Autodesk Fusion 360 part; units mm, degrees
sketch "Skizze1" plane through (0, 0, 0) normal (0, 0, 1) x (1, 0, 0)
  line L0 (-19, 19) -> (19, 19)
  line L1 (19, 19) -> (19, -19)
  line L2 (19, -19) -> (-19, -19)
  line L3 (-19, -19) -> (-19, 19)
  circle A0 centre (-14, 14) radius 1.175
  line L4 (0, 19) -> (0, -19) construction
  line L5 (-19, 0) -> (19, 0) construction
  circle A1 centre (14, 14) radius 1.175
  circle A2 centre (-14, -14) radius 1.175
  circle A3 centre (14, -14) radius 1.175
  circle A4 centre (-17, 17) radius 1
  circle A5 centre (17, 17) radius 1
  circle A6 centre (-17, -17) radius 1
  circle A7 centre (17, -17) radius 1
  circle A8 centre (-10, 0) radius 1
  circle A9 centre (10, 0) radius 1
  line L6 (-17, 16.5) -> (-6.5, 16.5) construction
  line L7 (-4.5, 16.5) -> (4.5, 16.5) construction
  line L8 (-4.5, 16) -> (4.5, 16)
  arc A10 (4.5, 16) -> (4.5, 17) centre (4.5, 16.5) ccw
  line L9 (4.5, 17) -> (-4.5, 17)
  arc A11 (-4.5, 17) -> (-4.5, 16) centre (-4.5, 16.5) ccw
  line L10 (-4.5, 16.5) -> (4.5, 16.5) construction
  line L11 (-6.5, 17) -> (-17, 17)
  arc A12 (-17, 17) -> (-17, 16) centre (-17, 16.5) ccw
  line L12 (-17, 16) -> (-6.5, 16)
  arc A13 (-6.5, 16) -> (-6.5, 17) centre (-6.5, 16.5) ccw
  line L13 (-6.5, 16.5) -> (-17, 16.5) construction
  line L14 (-19, 19) -> (19, -19) construction
  line L15 (6.5, 17) -> (17, 17)
  arc A14 (17, 16) -> (17, 17) centre (17, 16.5) ccw
  arc A15 (6.5, 17) -> (6.5, 16) centre (6.5, 16.5) ccw
  line L16 (17, 16) -> (6.5, 16)
  line L17 (-6.5, -17) -> (-17, -17)
  arc A16 (-17, -16) -> (-17, -17) centre (-17, -16.5) ccw
  arc A17 (-6.5, -17) -> (-6.5, -16) centre (-6.5, -16.5) ccw
  line L18 (4.5, -17) -> (-4.5, -17)
  arc A18 (-4.5, -16) -> (-4.5, -17) centre (-4.5, -16.5) ccw
  arc A19 (4.5, -17) -> (4.5, -16) centre (4.5, -16.5) ccw
  arc A20 (6.5, -16) -> (6.5, -17) centre (6.5, -16.5) ccw
  line L19 (6.5, -17) -> (17, -17)
  arc A21 (17, -17) -> (17, -16) centre (17, -16.5) ccw
  line L20 (17, -16) -> (6.5, -16)
  line L21 (-4.5, -16) -> (4.5, -16)
  line L22 (-17, -16) -> (-6.5, -16)
  line L23 (-17, -4.5) -> (-17, 4.5)
  arc A22 (-16, 4.5) -> (-17, 4.5) centre (-16.5, 4.5) ccw
  arc A23 (-17, -4.5) -> (-16, -4.5) centre (-16.5, -4.5) ccw
  line L24 (-16, 4.5) -> (-16, -4.5)
  arc A24 (17, 4.5) -> (16, 4.5) centre (16.5, 4.5) ccw
  line L25 (16, 4.5) -> (16, -4.5)
  arc A25 (16, -4.5) -> (17, -4.5) centre (16.5, -4.5) ccw
  line L26 (17, -4.5) -> (17, 4.5)
  line L27 (-17, 6.5) -> (-17, 17)
  arc A26 (-16, 17) -> (-17, 17) centre (-16.5, 17) ccw
  arc A27 (-17, 6.5) -> (-16, 6.5) centre (-16.5, 6.5) ccw
  line L28 (-16, 17) -> (-16, 6.5)
  arc A28 (-16, -6.5) -> (-17, -6.5) centre (-16.5, -6.5) ccw
  line L29 (-17, -6.5) -> (-17, -17)
  arc A29 (-17, -17) -> (-16, -17) centre (-16.5, -17) ccw
  line L30 (-16, -17) -> (-16, -6.5)
  arc A30 (17, 17) -> (16, 17) centre (16.5, 17) ccw
  line L31 (16, 17) -> (16, 6.5)
  arc A31 (16, 6.5) -> (17, 6.5) centre (16.5, 6.5) ccw
  line L32 (17, 6.5) -> (17, 17)
  line L33 (16, -17) -> (16, -6.5)
  arc A32 (17, -6.5) -> (16, -6.5) centre (16.5, -6.5) ccw
  arc A33 (16, -17) -> (17, -17) centre (16.5, -17) ccw
  line L34 (17, -6.5) -> (17, -17)
  dimension "d1" = 38
  dimension "d2" = 38
  dimension "d3" = 2.35
  dimension "d6" = 28
  dimension "d7" = 28
  dimension "d8" = 2
  dimension "d9" = 34
  dimension "d10" = 34
  dimension "d17" = 2
  dimension "d18" = 20
  dimension "d20" = 9
  dimension "d21" = 1
  dimension "d22" = 2
  dimension "d23" = 2.5
  dimension "d24" = 1
  dimension "d25" = 2
extrude "Extrusion1" add sketch "Skizze1" along normal blind 1.5
fillet "Abrundung1" radius 1 4 edges at (-16, -16, 0.75) (16, -16, 0.75) (16, 16, 0.75) (-16, 16, 0.75)
sketch "Skizze2" plane through (0, 0, 1.5) normal (0, 0, 1) x (-1, 0, 0)
  circle A0 centre (14, -14) radius 1.175
  circle A1 centre (-14, 14) radius 1.175
  circle A2 centre (14, 14) radius 1.175
  circle A3 centre (-14, -14) radius 1.175
  line L0 (19, 19) -> (-19, 19)
  line L1 (-19, 19) -> (-19, -19)
  line L2 (-19, -19) -> (19, -19)
  line L3 (19, -19) -> (19, 19)
  line L4 (8, -8) -> (-8, -8)
  line L5 (-8, -8) -> (-8, 8)
  line L6 (-8, 8) -> (8, 8)
  line L7 (8, 8) -> (8, -8)
  line L8 (0, -19) -> (0, 19) construction
  line L9 (19, 0) -> (-19, 0) construction
  circle A4 centre (10, 0) radius 1
  circle A5 centre (-10, 0) radius 1
  line L10 (-17, -4.5) -> (-17, 4.5)
  arc A6 (-16, 4.5) -> (-17, 4.5) centre (-16.5, 4.5) ccw
  line L11 (-16, 4.5) -> (-16, -4.5)
  arc A7 (-17, -4.5) -> (-16, -4.5) centre (-16.5, -4.5) ccw
  line L12 (-6.5, 16) -> (-15, 16)
  line L13 (-16, 15) -> (-16, 6.5)
  arc A8 (-17, 6.5) -> (-16, 6.5) centre (-16.5, 6.5) ccw
  line L14 (-17, 6.5) -> (-17, 16)
  arc A9 (-16, 17) -> (-17, 16) centre (-17, 17) ccw
  line L15 (-16, 17) -> (-6.5, 17)
  arc A10 (-6.5, 16) -> (-6.5, 17) centre (-6.5, 16.5) ccw
  arc A11 (-4.5, 17) -> (-4.5, 16) centre (-4.5, 16.5) ccw
  line L16 (-4.5, 17) -> (4.5, 17)
  arc A12 (4.5, 16) -> (4.5, 17) centre (4.5, 16.5) ccw
  line L17 (4.5, 16) -> (-4.5, 16)
  line L18 (-16, -6.5) -> (-16, -15)
  line L19 (-15, -16) -> (-6.5, -16)
  arc A13 (-6.5, -17) -> (-6.5, -16) centre (-6.5, -16.5) ccw
  line L20 (-6.5, -17) -> (-16, -17)
  arc A14 (-17, -16) -> (-16, -17) centre (-17, -17) ccw
  line L21 (-17, -16) -> (-17, -6.5)
  arc A15 (-16, -6.5) -> (-17, -6.5) centre (-16.5, -6.5) ccw
  line L22 (16, 6.5) -> (16, 15)
  line L23 (15, 16) -> (6.5, 16)
  arc A16 (6.5, 17) -> (6.5, 16) centre (6.5, 16.5) ccw
  line L24 (6.5, 17) -> (16, 17)
  arc A17 (17, 16) -> (16, 17) centre (17, 17) ccw
  line L25 (17, 16) -> (17, 6.5)
  arc A18 (16, 6.5) -> (17, 6.5) centre (16.5, 6.5) ccw
  arc A19 (17, 4.5) -> (16, 4.5) centre (16.5, 4.5) ccw
  line L26 (17, 4.5) -> (17, -4.5)
  arc A20 (16, -4.5) -> (17, -4.5) centre (16.5, -4.5) ccw
  line L27 (16, -4.5) -> (16, 4.5)
  arc A21 (4.5, -17) -> (4.5, -16) centre (4.5, -16.5) ccw
  line L28 (4.5, -17) -> (-4.5, -17)
  arc A22 (-4.5, -16) -> (-4.5, -17) centre (-4.5, -16.5) ccw
  line L29 (-4.5, -16) -> (4.5, -16)
  line L30 (6.5, -16) -> (15, -16)
  line L31 (16, -15) -> (16, -6.5)
  arc A23 (17, -6.5) -> (16, -6.5) centre (16.5, -6.5) ccw
  line L32 (17, -6.5) -> (17, -16)
  arc A24 (16, -17) -> (17, -16) centre (17, -17) ccw
  line L33 (16, -17) -> (6.5, -17)
  arc A25 (6.5, -16) -> (6.5, -17) centre (6.5, -16.5) ccw
  arc A26 (15, -16) -> (16, -15) centre (15, -15) ccw
  arc A27 (-16, -15) -> (-15, -16) centre (-15, -15) ccw
  arc A28 (-15, 16) -> (-16, 15) centre (-15, 15) ccw
  arc A29 (16, 15) -> (15, 16) centre (15, 15) ccw
  dimension "d13" = 16
  dimension "d14" = 16
extrude "Extrusion2" add sketch "Skizze2" along normal blind 1 contours L4 L5 L6 L7
sketch "Skizze3" plane through (0, 0, 0) normal (0, 0, -1) x (1, 0, 0)
  circle A0 centre (-14, 14) radius 1.175
  arc A1 (-4.5, -16) -> (-4.5, -17) centre (-4.5, -16.5) ccw
  line L0 (-4.5, -16) -> (4.5, -16)
  arc A2 (4.5, -17) -> (4.5, -16) centre (4.5, -16.5) ccw
  line L1 (4.5, -17) -> (-4.5, -17)
  circle A3 centre (-14, -14) radius 1.175
  circle A4 centre (14, -14) radius 1.175
  line L2 (-16, 15) -> (-16, 6.5)
  arc A5 (-17, 6.5) -> (-16, 6.5) centre (-16.5, 6.5) ccw
  line L3 (-17, 6.5) -> (-17, 16)
  arc A6 (-16, 17) -> (-17, 16) centre (-17, 17) ccw
  line L4 (-16, 17) -> (-6.5, 17)
  arc A7 (-6.5, 16) -> (-6.5, 17) centre (-6.5, 16.5) ccw
  line L5 (-6.5, 16) -> (-15, 16)
  circle A8 centre (-10, 0) radius 1
  line L6 (-15, -16) -> (-6.5, -16)
  arc A9 (-6.5, -17) -> (-6.5, -16) centre (-6.5, -16.5) ccw
  line L7 (-6.5, -17) -> (-16, -17)
  arc A10 (-17, -16) -> (-16, -17) centre (-17, -17) ccw
  line L8 (-17, -16) -> (-17, -6.5)
  arc A11 (-16, -6.5) -> (-17, -6.5) centre (-16.5, -6.5) ccw
  line L9 (-16, -6.5) -> (-16, -15)
  arc A12 (-16, 4.5) -> (-17, 4.5) centre (-16.5, 4.5) ccw
  line L10 (-16, 4.5) -> (-16, -4.5)
  arc A13 (-17, -4.5) -> (-16, -4.5) centre (-16.5, -4.5) ccw
  line L11 (-17, -4.5) -> (-17, 4.5)
  line L12 (15, 16) -> (6.5, 16)
  arc A14 (6.5, 17) -> (6.5, 16) centre (6.5, 16.5) ccw
  line L13 (6.5, 17) -> (16, 17)
  arc A15 (17, 16) -> (16, 17) centre (17, 17) ccw
  line L14 (17, 16) -> (17, 6.5)
  arc A16 (16, 6.5) -> (17, 6.5) centre (16.5, 6.5) ccw
  line L15 (16, 6.5) -> (16, 15)
  line L16 (16, -15) -> (16, -6.5)
  arc A17 (17, -6.5) -> (16, -6.5) centre (16.5, -6.5) ccw
  line L17 (17, -6.5) -> (17, -16)
  arc A18 (16, -17) -> (17, -16) centre (17, -17) ccw
  line L18 (16, -17) -> (6.5, -17)
  arc A19 (6.5, -16) -> (6.5, -17) centre (6.5, -16.5) ccw
  line L19 (6.5, -16) -> (15, -16)
  arc A20 (4.5, 16) -> (4.5, 17) centre (4.5, 16.5) ccw
  line L20 (4.5, 16) -> (-4.5, 16)
  arc A21 (-4.5, 17) -> (-4.5, 16) centre (-4.5, 16.5) ccw
  line L21 (-4.5, 17) -> (4.5, 17)
  circle A22 centre (14, 14) radius 1.175
  line L22 (17, 4.5) -> (17, -4.5)
  arc A23 (16, -4.5) -> (17, -4.5) centre (16.5, -4.5) ccw
  line L23 (16, -4.5) -> (16, 4.5)
  arc A24 (17, 4.5) -> (16, 4.5) centre (16.5, 4.5) ccw
  circle A25 centre (10, 0) radius 1
  line L24 (19, 19) -> (-19, 19)
  line L25 (-19, 19) -> (-19, -19)
  line L26 (-19, -19) -> (19, -19)
  line L27 (19, -19) -> (19, 19)
  arc A26 (-15, 16) -> (-16, 15) centre (-15, 15) ccw
  arc A27 (-16, -15) -> (-15, -16) centre (-15, -15) ccw
  arc A28 (16, 15) -> (15, 16) centre (15, 15) ccw
  arc A29 (15, -16) -> (16, -15) centre (15, -15) ccw
Work out the finished part from the listing and answer in its coordinate system (mm). A direction names the side the tool comes from. Give positions to 0.01 mm unless a question says otherwise; leave off trailing zeros. Loops run counter-clockwise (first coordinate to the right, second up) from the corner with the lowest first, then second, coordinate; pieces in that order, holes last. Notation, with made-up numbers: (82.5, 89) -> (132.5, 89) arc R9 cw to (132.5, 102) -> close; hole circle Ø8 at (40, -5). An arc over 180 degrees is marked (long way). Use a Markdown table: item, result. Add a question column.
1) Each of these flat-tipped pins is pushed along its axis until it touches: P1, Ø1.9, axis at x = -14, y = 14, coming from the -Z side; P2, Ø2.5, axis at x = 14, y = 14, coming from the +Z side. Where does it stop, or does it pass through?
2) The part is cut by section A-A, the plane y = 9. Determine the outline of the cut face in (x, z), plus the area to 3 significant figures.
3) Consider line 1 along Y through (x, z) = (2, 1.15); line 2 along Y through (x, z) = (10, 0.15); line 3 along Y through (x, z) = (14, 0.9) (3 decimals). Determine where each line is inside the solid, lowest interval first.
4) Which of the six approach directions +Z, -Z, +X, -X, +Y, -Y give full straight-line access (tool end or side, diameter ignored) to faces 5 (the flat face through (0, -8, 2)), 6 (the flat face through (17, 11, 1)), 7 (the flat face through (0, 8, 2))?
5) For a pull along Y with two mould halves and no side action, classify faces 1 (the flat face through (16, -11, 1)), 2 (the flat face through (17, -11, 1)), 3 (the flat face through (-8, 0, 2)), 4 (the flat face through (0, -19, 1)) as +Y half, -Y half, draft (parallel to the pull), parting line (faces both ways), or undercut.
6) The part is cut by section C-C, the plane y = 14. Determine the outline of the cut face in (x, z) (3 decimals).
Reported:
| question | item | result |
|---|---|---|
| 1 | P1 | passes through |
| 1 | P2 | stops at z = 1.5 |
| 2 | outline | (-19, 0) -> (-17, 0) -> (-17, 1.5) -> (-19, 1.5) -> close; (-16, 0) -> (16, 0) -> (16, 1.5) -> (-16, 1.5) -> close; (17, 0) -> (19, 0) -> (19, 1.5) -> (17, 1.5) -> close |
| 2 | area | 54.0 mm^2 |
| 3 | line 1 | y = -19 to -17, -16 to 16, 17 to 19 |
| 3 | line 2 | y = -19 to -17, -16 to -1, 1 to 16, 17 to 19 |
| 3 | line 3 | y = -19 to -17, -16 to -15.175, -12.825 to 12.825, 15.175 to 16, 17 to 19 |
| 4 | face 5 | +Z, +X, -X, -Y |
| 4 | face 6 | +Z, -Z |
| 4 | face 7 | +Z, +X, -X, +Y |
| 5 | face 1 | undercut |
| 5 | face 2 | undercut |
| 5 | face 3 | draft |
| 5 | face 4 | -Y half |
| 6 | outline | (-19, 0) -> (-17, 0) -> (-17, 1.5) -> (-19, 1.5) -> close; (-16, 0) -> (-15.175, 0) -> (-15.175, 1.5) -> (-16, 1.5) -> close; (-12.825, 0) -> (12.825, 0) -> (12.825, 1.5) -> (-12.825, 1.5) -> close; (15.175, 0) -> (16, 0) -> (16, 1.5) -> (15.175, 1.5) -> close; (17, 0) -> (19, 0) -> (19, 1.5) -> (17, 1.5) -> close |
